For this review, use the dimensioned drawing (mm, ordinates from the lowest corner) and the shaded views. Coordinates: 2 decimals unless noted, no trailing zeros. Loops run counter-clockwise (first coordinate to the right, second up) from the corner with the lowest first, then second, coordinate; pieces in that order, holes last. Notation, with made-up numbers: M 72,42.25 L 122,42.25 A31 ccw 122,76.25 Z; hole C -10.5,11 d5. An arc over 180 degrees is marked long. One line per item, written item: value.
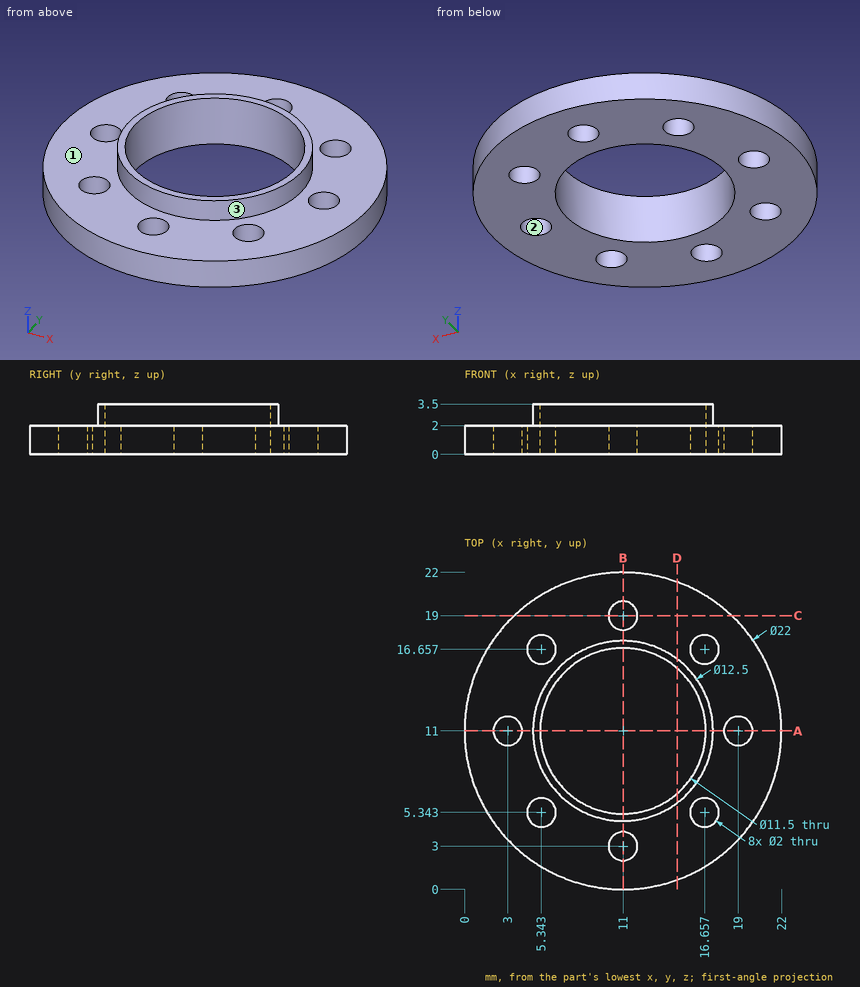
(1) To check wall thickness, follow L1, parallel to Y at x = 15.75, z = 1.4 (1 decimal); L2, parallel to Y at x = 15.75, z = 2.55; L3, parallel to Z at x = 15.5, y = 17.5. State the ranges of each line that lie inside material, in increasing order. Write a range as [from, to].
Checks:
L1: [1.1, 4.9], [5.8, 7.8], [14.2, 16.2], [17.1, 20.9]
L2: [6.94, 7.76], [14.24, 15.06]
L3: [0, 2]
(2) Insertion check: pin 1 Ø2.5 at (x, y) = (19, 11) entering from +Z; pin 2 Ø1 at (x, z) = (9, 2) entering from +Y; pin 3 Ø1 at (x, z) = (5, 1.5) entering from +Y. Each pin has a flat end and moves straight along its axis. Give the tip position at first contact, or say it passes through.
Checks:
pin 1: z = 2
pin 2: y = 21.9
pin 3: y = 20.53
(3) Draft analysis for pull direction Y (two halves, no side actions). For the marked faces 1, 2 and 3, state which applies: pulls with the +Y half, pulls with the -Y half, needs draft (parallel to the pull), parting line crosses it, or undercut.
Checks:
face 1: needs draft
face 2: undercut
face 3: parting line crosses it
(4) Add section A-A on y = 11. State the section outline as (x, z) points.
Checks:
outline: M 0,0 L 2,0 L 2,2 L 0,2 Z; M 4,0 L 5.25,0 L 5.25,3.5 L 4.75,3.5 L 4.75,2 L 4,2 Z; M 16.75,0 L 18,0 L 18,2 L 17.25,2 L 17.25,3.5 L 16.75,3.5 Z; M 20,0 L 22,0 L 22,2 L 20,2 Z
(5) Add section C-C on y = 19. State the section outline as (x, z) points.
Checks:
outline: M 3.45,0 L 10,0 L 10,2 L 3.45,2 Z; M 12,0 L 18.55,0 L 18.55,2 L 12,2 Z
(6) Add section D-D on x = 14.75. State the section outline as (y, z) points.
Checks:
outline: M 0.66,0 L 6.64,0 L 6.64,3.5 L 6,3.5 L 6,2 L 0.66,2 Z; M 15.36,0 L 21.34,0 L 21.34,2 L 16,2 L 16,3.5 L 15.36,3.5 Z
